from build123d import *

# Parameters (mm, degrees)
F1_DEPTH = 82.55
F2_W     = 44.45
F2_H     = 9.525
F3_DEPTH = 6.35
F4_DEPTH = 25.4
F5_R     = 3.175


with BuildPart() as f1:
    # F0 (on Front) → F1 (new body)
    with BuildSketch(Plane.XZ):
        with BuildLine():
            Line((-54.025357, 25.4), (-63.550357, 25.4))
            Line((-63.550357, 25.4), (-63.550357, -41.275))
            Line((-63.550357, -41.275), (136.474643, -41.275))
            Line((136.474643, -41.275), (136.474643, -22.225))
            Line((136.474643, -22.225), (12.649643, -22.225))
            ThreePointArc((12.649643, -22.225), (8.159515, -20.365128), (6.299643, -15.875))
            Line((6.299643, -15.875), (6.299643, 25.4))
            Line((6.299643, 25.4), (-3.225357, 25.4))
            Line((-3.225357, 25.4), (-22.275357, 6.35))
            Line((-22.275357, 6.35), (-22.275357, 0))
            Line((-22.275357, 0), (-34.975357, 0))
            Line((-34.975357, 0), (-34.975357, 6.35))
            Line((-34.975357, 6.35), (-54.025357, 25.4))
        make_face()
    extrude(amount=F1_DEPTH)

    # F2 (on face) → F3 (join)
    with BuildSketch(Plane.XY.offset(-22.225)):
        with BuildLine():
            Line((47.66174, -60.325), (47.66174, -50.8))
            ThreePointArc((47.66174, -50.8), (38.13674, -41.275), (47.66174, -31.75))
            Line((47.66174, -31.75), (47.66174, -22.225))
            ThreePointArc((47.66174, -22.225), (28.61174, -41.275), (47.66174, -60.325))
        make_face()
        with Locations((69.88674, -55.5625)):
            Rectangle(F2_W, F2_H)
        with BuildLine():
            ThreePointArc((92.11174, -31.75), (101.63674, -41.275), (92.11174, -50.8))
            Line((92.11174, -50.8), (92.11174, -60.325))
            ThreePointArc((92.11174, -60.325), (111.16174, -41.275), (92.11174, -22.225))
            Line((92.11174, -22.225), (92.11174, -31.75))
        make_face()
        with Locations((69.88674, -26.9875)):
            Rectangle(F2_W, F2_H)
    extrude(amount=F3_DEPTH)

    # F3_face (on face) → F4 (cut)
    with BuildSketch(Plane(origin=(69.88674, -41.275, -22.225), x_dir=(1, 0, 0), z_dir=(0, 0, 1))):
        with BuildLine():
            Line((-22.225, -9.525), (22.225, -9.525))
            ThreePointArc((22.225, -9.525), (31.75, 0), (22.225, 9.525))
            Line((22.225, 9.525), (-22.225, 9.525))
            ThreePointArc((-22.225, 9.525), (-31.75, 0), (-22.225, -9.525))
        make_face()
    extrude(amount=-F4_DEPTH, mode=Mode.SUBTRACT)

    # F5
    f5_edges = [f1.edges().sort_by_distance(p)[0] for p in [
        (69.88674, -60.325, -22.225),
    ]]
    fillet(f5_edges, radius=F5_R)


solid = f1.part
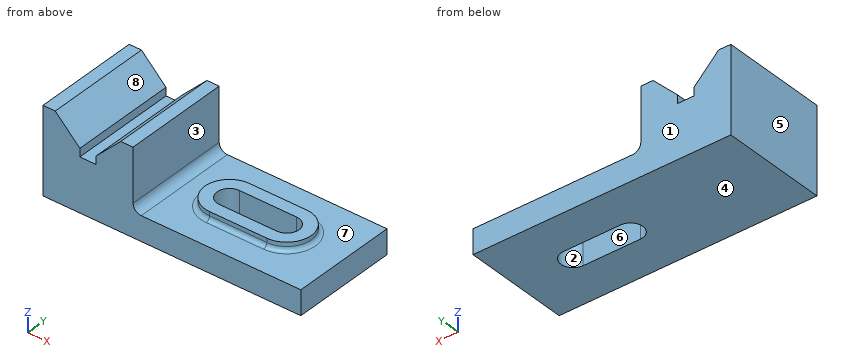
Here's how the part is built. I have some questions about the finished solid (model axes, mm). Face numbers are marked on the shaded views. A direction names the side the tool comes from. Give positions to 0.01 mm unless a question says otherwise; leave off trailing zeros. Loops run counter-clockwise (first coordinate to the right, second up) from the corner with the lowest first, then second, coordinate; pieces in that order, holes last. Notation, with made-up numbers: (30.25, -3.75) -> (73.25, -3.75) arc R19 cw to (73.25, 3.25) -> close; hole circle Ø7 at (87, 82). An arc over 180 degrees is marked (long way). One line per item, written item: value.
Q1. If I drill on line 1 along X through (y, z) = (-18.5, 5); line 2 along Z through (x, y) = (85.5, -55) (3 decimals); line 3 along Z through (x, y) = (128.5, -15) (3 decimals), over which ranges is the centre line in solid material (lowest first)?
Answers follow:
line 1: -63.55 to -34.98, -22.28 to 6.3
line 2: -41.275 to -15.875
line 3: -41.275 to -22.225
Q2. Suppose I cut it at D-D on z = 9. Please give me the cut outline in (x, y).
Answers follow:
outline: (-63.55, -82.55) -> (-37.63, -82.55) -> (-37.63, 0) -> (-63.55, 0) -> close; (-19.63, -82.55) -> (6.3, -82.55) -> (6.3, 0) -> (-19.63, 0) -> close
Q3. Suppose I cut it at B-B on z = -32.5. Please give me the cut outline in (x, y) (3 decimals).
Answers follow:
outline: (-63.55, -82.55) -> (136.475, -82.55) -> (136.475, 0) -> (-63.55, 0) -> close; hole (47.662, -50.8) -> (92.112, -50.8) arc R9.525 ccw to (92.112, -31.75) -> (47.662, -31.75) arc R9.525 ccw to start
Q4. On a 3-axis mill with a long thin cutter (end or side, diameter ignored), from which of +Z, -Z, +X, -X, +Y, -Y can I reach the whole of each face in a straight line? I mean the marked faces 4, 5, 6, 7 and 8. Say none if no direction works.
Answers follow:
face 4: -Z, +X, -X, +Y, -Y
face 5: +Z, -Z, -X, +Y, -Y
face 6: +Z, -Z
face 7: +Z
face 8: +Z, +Y, -Y
Q5. Suppose I cut it at A-A on x = 65. Please give me the cut outline in (y, z) (3 decimals).
Answers follow:
outline: (-82.55, -41.275) -> (-50.8, -41.275) -> (-50.8, -15.875) -> (-60.325, -15.875) -> (-60.325, -19.05) arc R3.175 cw to (-63.5, -22.225) -> (-82.55, -22.225) -> close; (-31.75, -41.275) -> (0, -41.275) -> (0, -22.225) -> (-19.05, -22.225) arc R3.175 cw to (-22.225, -19.05) -> (-22.225, -15.875) -> (-31.75, -15.875) -> close
Q6. We'd pull the mould along X, two halves only. Please class the marked faces 1, 2 and 3: pulls with the +X half, pulls with the -X half, needs draft (parallel to the pull), parting line crosses it, or undercut.
Answers follow:
face 1: needs draft
face 2: undercut
face 3: pulls with the +X half
Q7. I'm going to push flat-ended pins straight in: pin 1 Ø10 at (x, y) = (113.5, -22) entering from +Z (3 decimals); pin 2 Ø5 at (y, z) = (-62.5, -2.5) entering from +X; pin 3 Ø12.5 at (x, z) = (62.5, -23) entering from +Y; pin 4 Ø1 at (x, z) = (77.5, -18) entering from -Y (3 decimals). Where does each tip first touch, or does it pass through?
Answers follow:
pin 1: z = -22.225
pin 2: x = 6.3
pin 3: y = 0
pin 4: y = -60.325
Q8. Suppose I cut it at C-C on y = -77. Please give me the cut outline in (x, z) (3 decimals).
Answers follow:
outline: (-63.55, -41.275) -> (136.475, -41.275) -> (136.475, -22.225) -> (12.65, -22.225) arc R6.35 cw to (6.3, -15.875) -> (6.3, 25.4) -> (-3.225, 25.4) -> (-22.275, 6.35) -> (-22.275, 0) -> (-34.975, 0) -> (-34.975, 6.35) -> (-54.025, 25.4) -> (-63.55, 25.4) -> close
